For this review, use the dimensioned drawing (mm, ordinates from the lowest corner) and the shaded views. A direction names the side the tool comes from. Give positions to 0.01 mm unless a question says otherwise; leave off trailing zeros. Order: outer loops, then holes, each group sorted by start corner. A loop starts at its lowest first (then second) coordinate and runs counter-clockwise, first axis right, second up. Notation, with made-up numbers: M 84,-33 L 100,-33 A6 cw 100,-24 Z; hole C 21,10.5 d10. An arc over 180 degrees is marked long. One line per question, with ' | ' between items. Start each with the question number.
1. For the marked faces 1 and 2, list the 3-axis set-ups (+Z, -Z, +X, -X, +Y, -Y) from which the entire face can be reached by the end or side of a thin tool; tool diameter is ignored.
2. We need section B-B on x = 34. Write out the cut boundary in (y, z).
3. We need section C-C on x = 55. Write out the cut boundary in (y, z).
4. We need section D-D on y = 0.75. Write out the cut boundary in (x, z), then the cut area to 3 significant figures.
5. Wall thickness on L1, parallel to X at y = 4.75, z = 24.5 (1 decimal); L2, parallel to X at y = 1.25, z = 27 (1 decimal); L3, parallel to Y at x = 21, z = 18: over which ranges is each line inside the solid? List them lowest first.
6. We need section A-A on y = 5. Write out the cut boundary in (x, z) (1 decimal).
7. Insertion check: P1, Ø4.5, axis at x = 29, z = 25.4, coming from the -Y side; P2, Ø4, axis at y = 2.5, z = 6.5, coming from the -X side; P3, Ø4.5, axis at x = 55, z = 25.4, coming from the -Y side; P4, Ø1.5, axis at x = 6, y = 6, coming from the +Z side. Each pin has a flat end and moves straight along its axis. Give the tip position at first contact, or say it passes through.
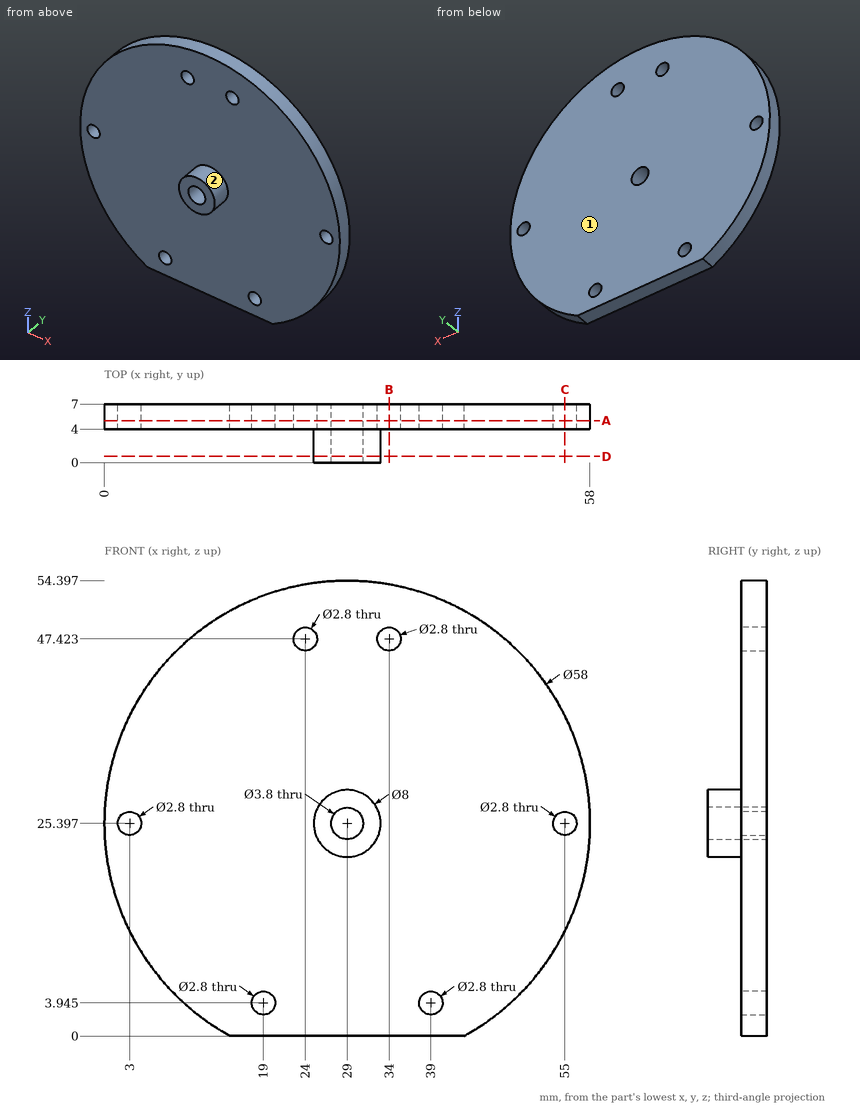
Entries:
1) face 1: +Z, -Z, +X, -X, +Y | face 2: -Y
2) outline: M 4,0 L 7,0 L 7,46.02 L 4,46.02 Z; M 4,48.82 L 7,48.82 L 7,53.96 L 4,53.96 Z
3) outline: M 4,12.55 L 7,12.55 L 7,24 L 4,24 Z; M 4,26.8 L 7,26.8 L 7,38.24 L 4,38.24 Z
4) outline: C 29,25.4 d8; hole C 29,25.4 d3.8 | area: 38.9 mm^2
5) L1: x = 0 to 1.9, 4.1 to 27.3, 30.7 to 53.9, 56.1 to 58 | L2: x = 25.3 to 28, 30 to 32.7 | L3: y = 4 to 7
6) outline: M 15,0 L 43,0 A29 ccw long Z; hole C 3,25.4 d2.8; hole C 19,3.9 d2.8; hole C 24,47.4 d2.8; hole C 29,25.4 d3.8; hole C 34,47.4 d2.8; hole C 39,3.9 d2.8; hole C 55,25.4 d2.8
7) P1: stops at y = 0 | P2: stops at x = 5.93 | P3: stops at y = 4 | P4: stops at z = 44
